Geometry check sheet. Reference: the model listing, model coordinates, mm. A direction names the side the tool comes from. Coordinates: 2 decimals unless noted, no trailing zeros. Write each loop counter-clockwise with the first axis right and the second up, starting at its lowest first coordinate (ties: lowest second). Pieces come first, ordered by that corner, then holes. Notation, with made-up numbers: M -35.75,51.5 L 10.25,51.5 A14 cw 10.25,74.5 Z; hole C 66,45.25 d3. An arc over 180 degrees is marked long. Write item = value, one per line. Start each with the question number.
```python
from build123d import *

# Parameters (mm, degrees)
SKETCH_1_W                     = 540
SKETCH_1_H                     = 570
EXTRUDE_1_DEPTH                = 90
CUT_EXTRUDE_1_REACH            = 619.191
SKETCH_2_W                     = 360
SKETCH_2_H                     = 20
SKETCH_2_W_2                   = 60
SKETCH_2_H_2                   = 10
SKETCH_2_W_3                   = 275
M30X2_0_1_D                    = 28
PATTERN_LINEAR_1_COUNT         = 4
PATTERN_LINEAR_1_PITCH         = 130
PATTERN_LINEAR_1_COUNT_DIR2    = 2
PATTERN_LINEAR_1_PITCH_DIR2    = 310
HOLE_WIZARD_M1_6_1_D           = 32
HOLE_WIZARD_M1_6_1_CBORE_D     = 72
HOLE_WIZARD_M1_6_1_CBORE_DEPTH = 30
PATTERN_LINEAR_2_COUNT         = 4
PATTERN_LINEAR_2_PITCH         = 105
HOLE_WIZARD_1_0_1_1_D          = 32
PATTERN_LINEAR_3_COUNT         = 4
PATTERN_LINEAR_3_PITCH         = 105
FILLET_1_R                     = 10
HOLE_WIZARD_M16_1_D            = 14
HOLE_WIZARD_M16_1_DEPTH        = 30
HOLE_WIZARD_M16_1_TIP          = 4.206024333
CHAMFER_1_SIZE                 = 5


with BuildPart() as part:
    # 草图1 → 凸台-拉伸1 (new body)
    with BuildSketch(Plane(origin=(0, 0, 0), x_dir=(1, 0, 0), z_dir=(0, 1, 0))):
        Rectangle(SKETCH_1_W, SKETCH_1_H)
    extrude(amount=-EXTRUDE_1_DEPTH)

    # 草图2 → 切除-拉伸1 (cut, up to next)
    with BuildSketch(Plane.ZY.offset(270), mode=Mode.PRIVATE) as cut_extrude_1_sk1:
        with Locations((-105, -10)):
            Rectangle(SKETCH_2_W, SKETCH_2_H)
    cut_extrude_1_tool1 = extrude(cut_extrude_1_sk1.sketch, amount=-CUT_EXTRUDE_1_REACH, mode=Mode.PRIVATE) & part.part
    # 草图2 → 切除-拉伸1 (cut, up to next)
    with BuildSketch(Plane.ZY.offset(270), mode=Mode.PRIVATE) as cut_extrude_1_sk2:
        with Locations((-255, -85)):
            Rectangle(SKETCH_2_W_2, SKETCH_2_H_2)
    cut_extrude_1_tool2 = extrude(cut_extrude_1_sk2.sketch, amount=-CUT_EXTRUDE_1_REACH, mode=Mode.PRIVATE) & part.part
    # 草图2 → 切除-拉伸1 (cut, up to next)
    with BuildSketch(Plane.ZY.offset(270), mode=Mode.PRIVATE) as cut_extrude_1_sk3:
        with Locations((92.5, -85)):
            Rectangle(SKETCH_2_W_3, SKETCH_2_H_2)
    cut_extrude_1_tool3 = extrude(cut_extrude_1_sk3.sketch, amount=-CUT_EXTRUDE_1_REACH, mode=Mode.PRIVATE) & part.part
    add(cut_extrude_1_tool1.solids().sort_by_distance((-270, -10, -105))[0], mode=Mode.SUBTRACT)
    add(cut_extrude_1_tool2.solids().sort_by_distance((-270, -85, -255))[0], mode=Mode.SUBTRACT)
    add(cut_extrude_1_tool3.solids().sort_by_distance((-270, -85, 92.5))[0], mode=Mode.SUBTRACT)

    # M30x2.0 螺纹孔1 (through all)
    with Locations(Plane(origin=(180, -20, 50), x_dir=(0, 0, 1), z_dir=(0, 1, 0))):
        with Locations((0, 0)):
            m30x2_0_1 = Hole(M30X2_0_1_D / 2)

    # 阵列(线性)1: M30x2.0 _1 4 × 2
    with Locations(*[(-i * PATTERN_LINEAR_1_PITCH, 0, -j * PATTERN_LINEAR_1_PITCH_DIR2) for i in range(PATTERN_LINEAR_1_COUNT) for j in range(PATTERN_LINEAR_1_COUNT_DIR2) if (i, j) != (0, 0)]):
        add(m30x2_0_1, mode=Mode.SUBTRACT)

    # M1.6 六角头螺栓的柱形沉头孔1 (through all)
    with Locations(Plane(origin=(-205, -20, -192.080967971), x_dir=(0, 0, 1), z_dir=(0, 1, 0))):
        with Locations((0, 0)):
            hole_wizard_m1_6_1 = CounterBoreHole(HOLE_WIZARD_M1_6_1_D / 2, HOLE_WIZARD_M1_6_1_CBORE_D / 2, HOLE_WIZARD_M1_6_1_CBORE_DEPTH)

    # 阵列(线性)2: M1.6 六角头螺栓的柱形沉头孔1 ×4
    with Locations(*[(i * PATTERN_LINEAR_2_PITCH, 0, 0) for i in range(1, PATTERN_LINEAR_2_COUNT)]):
        add(hole_wizard_m1_6_1, mode=Mode.SUBTRACT)

    # Ø1.0 (1) 直径孔1 (through all)
    with Locations(Plane(origin=(-205, 0, 257.5), x_dir=(0, 0, 1), z_dir=(0, 1, 0))):
        with Locations((0, 0)):
            hole_wizard_1_0_1_1 = Hole(HOLE_WIZARD_1_0_1_1_D / 2)

    # 阵列(线性)3: Ø1.0 (1) 直径孔1 ×4
    with Locations(*[(i * PATTERN_LINEAR_3_PITCH, 0, 0) for i in range(1, PATTERN_LINEAR_3_COUNT)]):
        add(hole_wizard_1_0_1_1, mode=Mode.SUBTRACT)

    # 圆角1
    fillet_1_edges = [part.edges().sort_by_distance(p)[0] for p in [
        (0, -80, -45),
        (0, -80, 230),
        (0, -80, -225),
    ]]
    fillet(fillet_1_edges, radius=FILLET_1_R - 0.0001)  # a hair under: the kernel refuses the full size

    # M16 螺纹孔1
    with Locations(Plane(origin=(-150, -48, -285), x_dir=(-1, 0, 0), z_dir=(0, 0, -1))):
        with Locations((0, 0), (-300, 0)):
            Hole(HOLE_WIZARD_M16_1_D / 2, depth=HOLE_WIZARD_M16_1_DEPTH)
            with Locations((0, 0, -(HOLE_WIZARD_M16_1_DEPTH + HOLE_WIZARD_M16_1_TIP / 2))):  # 118° drill point
                Cone(0, HOLE_WIZARD_M16_1_D / 2, HOLE_WIZARD_M16_1_TIP, mode=Mode.SUBTRACT)

    # 倒角1
    chamfer_1_edges = [part.edges().sort_by_distance(p)[0] for p in [
        (270, -50, -285),
        (-270, -50, -285),
        (270, -45, 285),
        (-270, -45, 285),
    ]]
    chamfer(chamfer_1_edges, length=CHAMFER_1_SIZE)


solid = part.part
```
Q1. Cross-section at C-C on z = -24.5. Enter the section's corners in (x, y).
Q2. Cross-section at A-A on x = 180. Count the separate pieces of the cut face and the enclosed holes in it, and give its area (3 significant figures).
Q3. Draft check along Z on faces 4 (the face through (193.88, -50.42, 51.82)), 5 (the face through (-4, 0, 179)), 6 (the face through (-4, -10, 75)). Enter one of: pulls with the +Z half, pulls with the -Z half, needs draft (parallel to the pull), parting line crosses it, or undercut.
Q4. Gauge pin test, flat ends, axial feed: pin 1 (1 mm diameter, centred on x = 53, z = -22, fed in from +Y); pin 2 (4 mm diameter, centred on x = -82, z = 15.5, fed in from -Y); pin 3 (8 mm diameter, centred on x = 155, y = -14.5, fed in from -Z). Record the tip position at first contact, or that the pin passes through.
Q5. Scan lines: L1, parallel to X at y = -31.5, z = 257.5; L2, parallel to X at y = -53, z = 50; L3, parallel to Z at x = -191, y = -21. Record each from-to range of solid material in increasing order.
Q6. Set-up check for faces 1 (the face through (-180.669, -34.79, -218.614)), 2 (the face through (-4, -80, -260)), 3 (the face through (-4, -90, 275)): record each of +Z, -Z, +X, -X, +Y, -Y from which the full face is reachable in a straight line by a thin tool's end or side.
Values found:
q1.outline = M -270,-80 L 270,-80 L 270,-20 L -270,-20 Z
q2.separate_pieces = 3
q2.enclosed_holes = 0
q2.area = 37,500 mm²
q3.face_4 = undercut
q3.face_5 = needs draft
q3.face_6 = pulls with the -Z half
q4.pin_1 = -20
q4.pin_2 = -80
q4.pin_3 = 75
q5.L1 = -270 to -221, -189 to -116, -84 to -11, 21 to 94, 126 to 270
q5.L2 = -270 to -224, -196 to -94, -66 to 36, 64 to 166, 194 to 270
q5.L3 = -285 to -225.25, -158.91 to 249.75, 265.25 to 285
q6.face_1 = +Y
q6.face_2 = -Z, +X, -X, -Y
q6.face_3 = +Z, -Z, +X, -X, -Y
